from build123d import *

# Parameters (mm, degrees)
CHAMFER1_SIZE = 0.32
CHAMFER2_SIZE = 0.4


with BuildPart() as part:
    # Sketch1 → Revolve1 (revolve)
    with BuildSketch(Plane(origin=(0, 0, 0), x_dir=(0, 0, -1), z_dir=(1, 0, 0))):
        with BuildLine():
            Line((-8, 0), (-8, 8))
            Line((-8, 8), (-0.05, 8))
            ThreePointArc((-0.05, 8), (-0.014644661, 7.985355339), (0, 7.95))
            Line((0, 7.95), (0, 4.447213595))
            ThreePointArc((0, 4.447213595), (-0.0127322, 4.413880262), (-0.044444444, 4.397523196))
            ThreePointArc((-0.044444444, 4.397523196), (-0.399380319, 3.977743298), (0, 3.6))
            Line((0, 3.6), (0.8, 3.6))
            Line((0.8, 3.6), (0.8, 4))
            Line((0.8, 4), (12, 4))
            Line((12, 4), (12, 0))
            Line((12, 0), (-8, 0))
        make_face()
    revolve(axis=Axis((0, 0, 12.7), (0, 0, -1)))

    # Chamfer1
    chamfer1_edges = [part.edges().sort_by_distance(p)[0] for p in [
        (0, -8, 8),
    ]]
    chamfer(chamfer1_edges, length=CHAMFER1_SIZE)

    # Chamfer2
    chamfer2_edges = [part.edges().sort_by_distance(p)[0] for p in [
        (0, -4, -12),
    ]]
    chamfer(chamfer2_edges, length=CHAMFER2_SIZE)


solid = part.part
Work out the finished part from the listing and answer in its coordinate system (mm). A direction names the side the tool comes from. Give positions to 0.01 mm unless a question says otherwise; leave off trailing zeros. Loops run counter-clockwise (first coordinate to the right, second up) from the corner with the lowest first, then second, coordinate; pieces in that order, holes last. Notation, with made-up numbers: (69.5, 75.25) - (93.5, 75.25) arc R8 cw to (93.5, 85.25) - close; hole circle Ø9 at (64.25, 72). An arc over 180 degrees is marked (long way). Answer in a Markdown table with one row per item.
(1) A tool of negligible diameter and unlimited length cuts with its end or side. For faces 1 (the face through (-7.81, -1.73, 3.81)), 2 (the face through (-3.905, -0.867, -6.276)), from which of +Z, -Z, +X, -X, +Y, -Y can it reach the whole face along a straight path? Write none if from no direction.
Results list:
| item | result |
|---|---|
| face 1 | +Z, -Z |
| face 2 | -Z |
(2) Flat-ended cylindrical pins translate along their axes: pin 1 Ø5 at (x, z) = (-3.5, 3.5) entering from +Y; pin 2 Ø6 at (x, z) = (-4.5, -3.5) entering from +Y; pin 3 Ø2 at (y, z) = (-6.5, 1.5) entering from +X. Find the tip coordinate at first contact, or state that the pin passes through.
Results list:
| item | result |
|---|---|
| pin 1 | stops at y = 7.94 |
| pin 2 | stops at y = 3.71 |
| pin 3 | stops at x = 5.81 |
(3) Section C-C (z = -6) is taken. Give the vertices of the cut face in (x, y).
Results list:
| item | result |
|---|---|
| outline | circle Ø8 at (0, 0) |
(4) Section D-D (z = 1.5) is taken. Give the vertices of the cut face in (x, y).
Results list:
| item | result |
|---|---|
| outline | circle Ø16 at (0, 0) |
(5) Section A-A (y = 0) is taken. Give the vertices of the cut face in (x, z), and give its area (3 significant figures).
Results list:
| item | result |
|---|---|
| outline | (-8, 0.05) arc R0.05 ccw to (-7.95, 0) - (-4.45, 0) arc R0.05 ccw to (-4.4, 0.04) arc R0.4 cw to (-3.6, 0) - (-3.6, -0.8) - (-4, -0.8) - (-4, -11.6) - (-3.6, -12) - (3.6, -12) - (4, -11.6) - (4, -0.8) - (3.6, -0.8) - (3.6, 0) arc R0.4 cw to (4.4, 0.04) arc R0.05 ccw to (4.45, 0) - (7.95, 0) arc R0.05 ccw to (8, 0.05) - (8, 7.68) - (7.68, 8) - (-7.68, 8) - (-8, 7.68) - close |
| area | 223 mm² |
(6) For a pull along Z with two mould halves and no side action, classify faces 3 (the face through (0, 0, 8)), 4 (the face through (1.081, 3.434, -0.406)), 5 (the face through (0, 0, -12)) as pulls with the +Z half, pulls with the -Z half, needs draft (parallel to the pull), parting line crosses it, or undercut.
Results list:
| item | result |
|---|---|
| face 3 | pulls with the +Z half |
| face 4 | undercut |
| face 5 | pulls with the -Z half |
(7) Consider L1, parallel to Z at x = -7.25, y = -0.5; L2, parallel to X at y = -3, z = -5; L3, parallel to X at y = -3.25, z = -10.25. Determine where each line is inside the solid, lowest interval first. Write a range as [from, to].
Results list:
| item | result |
|---|---|
| L1 | z = [0, 8] |
| L2 | x = [-2.65, 2.65] |
| L3 | x = [-2.33, 2.33] |
